from build123d import *

# Parameters (mm, degrees)
SKETCH_1_W          = 14.55
SKETCH_1_H          = 11.7
EXTRUDE_1_DEPTH     = 1
SKETCH_2_W          = 14.45
SKETCH_2_H          = 8.4
CUT_EXTRUDE_1_DEPTH = 0.05
SKETCH_3_W          = 14.55
SKETCH_3_H          = 16.9
EXTRUDE_2_DEPTH     = 3


with BuildPart() as part:
    # Эскиз1 → Бобышка-Вытянуть1 (new body)
    with BuildSketch(Plane.XY):
        Rectangle(SKETCH_1_W, SKETCH_1_H)
    extrude(amount=EXTRUDE_1_DEPTH)

    # Эскиз2 → Вырез-Вытянуть1 (cut)
    with BuildSketch(Plane.XY.offset(1)):
        with Locations((0, 1.6)):
            Rectangle(SKETCH_2_W, SKETCH_2_H)
    extrude(amount=-CUT_EXTRUDE_1_DEPTH, mode=Mode.SUBTRACT)

    # Эскиз3 → Бобышка-Вытянуть2 (add)
    with BuildSketch(Plane(origin=(0, 0, 0), x_dir=(-1, 0, 0), z_dir=(0, 0, -1))):
        with Locations((0, 0.9)):
            Rectangle(SKETCH_3_W, SKETCH_3_H)
    extrude(amount=EXTRUDE_2_DEPTH)


solid = part.part
Geometry check sheet. Reference: the model listing, model coordinates, mm. A direction names the side the tool comes from. Round coordinates to 2 decimals unless told otherwise and drop trailing zeros. Write each loop counter-clockwise with the first axis right and the second up, starting at its lowest first coordinate (ties: lowest second). Pieces come first, ordered by that corner, then holes.
Item 1: Material ranges on line 1 along Z through (x, y) = (-4.25, 2.5); line 2 along Z through (x, y) = (-0.75, 8.75); line 3 along Y through (x, z) = (-1.75, 0.15), recorded low to high.
Determined:
line 1: z = -3 to 0.95
line 2: z = -3 to 0
line 3: y = -5.85 to 5.85
Item 2: Section check B-B (y = 7). Record the boundary of the cut face in (x, z) (3 decimals).
Determined:
outline: (-7.275, -3) - (7.275, -3) - (7.275, 0) - (-7.275, 0) - close
Item 3: Section check A-A (x = 4). Record the boundary of the cut face in (y, z).
Determined:
outline: (-7.55, -3) - (9.35, -3) - (9.35, 0) - (5.85, 0) - (5.85, 1) - (5.8, 1) - (5.8, 0.95) - (-2.6, 0.95) - (-2.6, 1) - (-5.85, 1) - (-5.85, 0) - (-7.55, 0) - close
Item 4: Go/stop test with flat-tipped pins: pin 1 Ø0.5 at (x, y) = (-2.5, -6.5) entering from +Z; pin 2 Ø0.5 at (x, z) = (0, 0.5) entering from +Y. Record where each tip stops, or that it passes through.
Determined:
pin 1: stops at z = 0
pin 2: stops at y = 5.85
Item 5: Access from +Z, -Z, +X, -X, +Y, -Y to the whole of each face (thin tool, end or side, straight path). Record for faces 1 (the face through (7.275, 1, -1)), 2 (the face through (-0.1, -5.85, 0.5)), 3 (the face through (0, -7.55, -1)), 4 (the face through (0, 2, 0.95)), 5 (the face through (0, 8, 0)).
Determined:
face 1: +Z, -Z, +X, +Y, -Y
face 2: +Z, +X, -X, -Y
face 3: +Z, -Z, +X, -X, -Y
face 4: +Z
face 5: +Z, +X, -X, +Y
